from build123d import *

# Parameters (mm, degrees)
F0_W          = 76.2
F0_H          = 76.2
F0_W_2        = 63.5
F0_H_2        = 63.5
F1_DEPTH      = 762
F2_R          = 19.05
F3_DEPTH      = 25.4
F3_DEPTH_BACK = 101.6
F4_R          = 12.7
F5_DEPTH      = 127.001


with BuildPart() as f1:
    # F0 (on Top) → F1 (new body)
    with BuildSketch(Plane.XY):
        Rectangle(F0_W, F0_H)
        Rectangle(F0_W_2, F0_H_2, mode=Mode.SUBTRACT)
    extrude(amount=F1_DEPTH)

    # F2 (on face) → F3 (join, two sides)
    with BuildSketch(Plane.YZ.offset(38.1)) as f3_sk:
        with Locations((0, 76.2)):
            Circle(F2_R)
    extrude(amount=F3_DEPTH)
    extrude(f3_sk.sketch, amount=-F3_DEPTH_BACK)

    # F4 (on face) → F5 (cut, through all)
    with BuildSketch(Plane(origin=(-63.5, 0, 0), x_dir=(0, -1, 0), z_dir=(-1, 0, 0))):
        with Locations((0, 76.2)):
            Circle(F4_R)
    extrude(amount=-F5_DEPTH, mode=Mode.SUBTRACT)


solid = f1.part
Verification items for the finished model (mm, model axes). A direction names the side the tool comes from. Round coordinates to 2 decimals unless told otherwise and drop trailing zeros. Loops run counter-clockwise (first coordinate to the right, second up) from the corner with the lowest first, then second, coordinate; pieces in that order, holes last. Notation, with made-up numbers: M 18,-9.75 L 36,-9.75 A32 cw 36,29.25 Z; hole C -28.75,24 d5. An arc over 180 degrees is marked long. Write each question's results on one line, items separated by ' | '.
1) Section check C-C on y = 0. Record the boundary of the cut face in (x, z), then the cut area to 3 significant figures.
Checks:
outline: M -63.5,57.15 L -38.1,57.15 L -38.1,0 L -31.75,0 L -31.75,57.15 L 31.75,57.15 L 31.75,0 L 38.1,0 L 38.1,57.15 L 63.5,57.15 L 63.5,63.5 L -63.5,63.5 Z; M -63.5,88.9 L 63.5,88.9 L 63.5,95.25 L 38.1,95.25 L 38.1,762 L 31.75,762 L 31.75,95.25 L -31.75,95.25 L -31.75,762 L -38.1,762 L -38.1,95.25 L -63.5,95.25 Z | area: 10,800 mm2
2) Section check D-D on z = 344.5. Record the boundary of the cut face in (x, y), then the cut area to 3 significant figures.
Checks:
outline: M -38.1,-38.1 L 38.1,-38.1 L 38.1,38.1 L -38.1,38.1 Z; hole M -31.75,-31.75 L 31.75,-31.75 L 31.75,31.75 L -31.75,31.75 Z | area: 1,770 mm2
3) Mould release check, pull along X, two halves, no side actions. Record for faces 1 (the flat face through (-63.5, 12.4, 72.2)), 2 (the flat face through (0, 31.75, 376)), 3 (the flat face through (-1, 38.1, 376)), 4 (the flat face through (38.1, -1, 376)): released by +X, released by -X, zero draft, split by the parting line, or undercut.
Checks:
face 1: released by -X | face 2: undercut | face 3: zero draft | face 4: released by +X
4) Scan lines: L1, parallel to Y at x = -27, z = 76; L2, parallel to Y at x = 31.5, z = 342.5. Record each from-to range of solid material in increasing order. Write a range as from..to.
Checks:
L1: y = -38.1..-31.75, -19.05..-12.7, 12.7..19.05, 31.75..38.1 | L2: y = -38.1..-31.75, 31.75..38.1
5) Section check B-B on z = 76.2. Record the boundary of the cut face in (x, y), then the cut area to 3 significant figures.
Checks:
outline: M -63.5,-19.05 L -38.1,-19.05 L -38.1,-38.1 L 38.1,-38.1 L 38.1,-19.05 L 63.5,-19.05 L 63.5,-12.7 L -63.5,-12.7 Z; M -63.5,12.7 L 63.5,12.7 L 63.5,19.05 L 38.1,19.05 L 38.1,38.1 L -38.1,38.1 L -38.1,19.05 L -63.5,19.05 Z; hole M -31.75,-31.75 L 31.75,-31.75 L 31.75,-19.05 L -31.75,-19.05 Z; hole M -31.75,19.05 L 31.75,19.05 L 31.75,31.75 L -31.75,31.75 Z | area: 2,900 mm2
6) Section check A-A on x = -19.5. Record the boundary of the cut face in (y, z).
Checks:
outline: M -38.1,0 L -31.75,0 L -31.75,762 L -38.1,762 Z; C 0,76.2 d38.1; M 31.75,0 L 38.1,0 L 38.1,762 L 31.75,762 Z; hole C 0,76.2 d25.4
7) Gauge pin test, flat ends, axial feed: P1, Ø8, axis at y = -7, z = 297.5, coming from the -X side; P2, Ø6, axis at x = -39.5, y = 2, coming from the +Z side; P3, Ø1.5, axis at x = 50.5, y = 21, coming from the +Z side; P4, Ø1, axis at y = -17.5, z = 445.5, coming from the +X side. Record the tip position at first contact, or that the pin passes through.
Checks:
P1: stops at x = -38.1 | P2: stops at z = 762 | P3: passes through | P4: stops at x = 38.1
8) Access from +Z, -Z, +X, -X, +Y, -Y to the whole of each face (thin tool, end or side, straight path). Record for faces 5 (the cylindrical face through (-50.622, -2.48, 95.088)), 6 (the cylindrical face through (50.622, -2.48, 95.088)), 7 (the flat face through (0, -31.75, 376)), 8 (the cylindrical face through (0.445, -2.48, 95.088)).
Checks:
face 5: -X | face 6: +X | face 7: +Z, -Z | face 8: none
